from build123d import *

# Parameters (mm, degrees)
SKETCH1_W           = 33.5
SKETCH1_H           = 16
BOSS_EXTRUDE1_DEPTH = 32
SKETCH2_W           = 23.5
SKETCH2_H           = 16
CUT_EXTRUDE1_DEPTH  = 12
SKETCH4_R           = 0.5
BOSS_EXTRUDE2_DEPTH = 0.5
FILLET1_R           = 0.5
SKETCH6_W           = 16
SKETCH6_H           = 2
BOSS_EXTRUDE3_DEPTH = 75.5
SKETCH7_W           = 5
SKETCH7_H           = 5.252635659
CUT_EXTRUDE2_DEPTH  = 9
SKETCH8_R           = 0.8
CUT_EXTRUDE3_DEPTH  = 8
SKETCH9_R           = 0.5
SKETCH9_R_2         = 2
CUT_EXTRUDE4_DEPTH  = 8
FILLET2_R           = 30


with BuildPart() as part:
    # Sketch1 → Boss-Extrude1 (new body)
    with BuildSketch(Plane(origin=(0, 0, 0), x_dir=(1, 0, 0), z_dir=(0, 1, 0))):
        Rectangle(SKETCH1_W, SKETCH1_H)
    extrude(amount=BOSS_EXTRUDE1_DEPTH)

    # Sketch2 → Cut-Extrude1 (cut)
    with BuildSketch(Plane(origin=(0, 32, 0), x_dir=(1, 0, 0), z_dir=(0, 1, 0))):
        Rectangle(SKETCH2_W, SKETCH2_H)
    extrude(amount=-CUT_EXTRUDE1_DEPTH, mode=Mode.SUBTRACT)

    # Sketch4 → Boss-Extrude2 (add)
    with BuildSketch(Plane(origin=(0, 0, 0), x_dir=(-1, 0, 0), z_dir=(0, -1, 0))):
        with Locations(Location((15.81324072, -7.12248893, 0), (0, 0, 270))):
            Circle(SKETCH4_R)
        with Locations(Location((-15.868829232, -7.12248893, 0), (0, 0, 270))):
            Circle(SKETCH4_R)
        with Locations(Location((-15.868829232, 7.12248893, 0), (0, 0, 270))):
            Circle(SKETCH4_R)
        with Locations(Location((15.81324072, 7.12248893, 0), (0, 0, 270))):
            Circle(SKETCH4_R)
    extrude(amount=BOSS_EXTRUDE2_DEPTH)

    # Fillet1
    fillet1_edges = [part.edges().sort_by_distance(p)[0] for p in [
        (-15.81324072, -0.5, 6.62248893),
        (15.868829232, -0.5, 6.62248893),
        (15.868829232, -0.5, -7.62248893),
        (-15.81324072, -0.5, -7.62248893),
    ]]
    fillet(fillet1_edges, radius=FILLET1_R - 0.0001)  # a hair under: the kernel refuses the full size

    # Sketch6 → Boss-Extrude3 (add)
    with BuildSketch(Plane.ZY.offset(16.75)):
        with Locations((0, 31)):
            Rectangle(SKETCH6_W, SKETCH6_H)
    extrude(amount=BOSS_EXTRUDE3_DEPTH)

    # Sketch7 → Cut-Extrude2 (cut)
    with BuildSketch(Plane(origin=(0, 32, 0), x_dir=(1, 0, 0), z_dir=(0, 1, 0))):
        with Locations((14.25, -5.373682171)):
            Rectangle(SKETCH7_W, SKETCH7_H)
    extrude(amount=-CUT_EXTRUDE2_DEPTH, mode=Mode.SUBTRACT)

    # Sketch8 → Cut-Extrude3 (cut)
    with BuildSketch(Plane.XY):
        with Locations((13.65, 26)):
            Circle(SKETCH8_R)
        with Locations((-13.65, 26)):
            Circle(SKETCH8_R)
    extrude(amount=-CUT_EXTRUDE3_DEPTH, mode=Mode.SUBTRACT)

    # Sketch9 → Cut-Extrude4 (cut)
    with BuildSketch(Plane(origin=(0, 32, 0), x_dir=(1, 0, 0), z_dir=(0, 1, 0))):
        with Locations(Location((-88.515974664, 6.5, 0), (0, 0, 270))):
            Circle(SKETCH9_R)
        with Locations(Location((-75.25, 0, 0), (0, 0, 270))):
            Circle(SKETCH9_R)
        with Locations(Location((-88.515974664, -6.5, 0), (0, 0, 270))):
            Circle(SKETCH9_R)
        with Locations(Location((-88.515974664, 0, 0), (0, 0, 270))):
            Circle(SKETCH9_R_2)
    extrude(amount=-CUT_EXTRUDE4_DEPTH, mode=Mode.SUBTRACT)

    # Fillet2
    fillet2_edges = [part.edges().sort_by_distance(p)[0] for p in [
        (-16.75, 30, 0),
    ]]
    fillet(fillet2_edges, radius=FILLET2_R - 0.0001)  # a hair under: the kernel refuses the full size


solid = part.part
Input: part model. Units: mm. Frame: model coordinates. A direction names the side the tool comes from. Coordinates: 2 decimals unless noted, no trailing zeros. Loops run counter-clockwise (first coordinate to the right, second up) from the corner with the lowest first, then second, coordinate; pieces in that order, holes last.
(1) Material intervals for probe 1 along X at (y, z) = (31.3, 0); probe 2 along X at (y, z) = (31.5, -6.5); probe 3 along X at (y, z) = (31, 6.5), sorted ascending.
(2) Pull-direction query (X, two-part tool) for faces 1 (the face through (0, 20, 0)), 2 (the face through (-25.771, 21.445, 0.112)), 3 (the face through (14, 32, -3)); classes: released by +X, released by -X, zero draft, split by the parting line, or undercut.
(3) First-contact query: pin 1 Ø8 at (y, z) = (27.5, -3.5) entering from -X; pin 2 Ø5 at (x, z) = (-88.52, 0) entering from -Y; pin 3 Ø1 at (x, y) = (13.65, 26) entering from -Z; pin 4 Ø4 at (y, z) = (24.5, 1) entering from -X. Flat tips, straight axial feed; report the tip coordinate or a pass-through.
(4) Section C-C on y = 18.5. Return the cut outline in (x, z), then the cut area to 3 significant figures.
(5) Set-up query: faces 4 (the face through (14, 23, 5)), 5 (the face through (11.75, 26, -2)), 6 (the face through (-9, 17, -8)), 7 (the face through (16.75, 16, 0)), 8 (the face through (-69, 30, 0)). Return all of +Z, -Z, +X, -X, +Y, -Y with unobstructed straight access to the full face (end or side cutting, diameter ignored); none if empty.
(6) Section B-B on x = -72. Return the cut outline in (y, z).
Data:
1. probe 1: x = -92.25 to -90.52, -86.52 to -75.75, -74.75 to -11.75, 11.75 to 16.75
1. probe 2: x = -92.25 to -89.02, -88.02 to -11.75, 11.75 to 16.75
1. probe 3: x = -92.25 to -89.02, -88.02 to -11.75
2. face 1: undercut
2. face 2: released by -X
2. face 3: zero draft
3. pin 1: stops at x = -92.25
3. pin 2: stops at y = 30
3. pin 3: stops at z = 0
3. pin 4: stops at x = -32.69
4. outline: (-23.13, -8) - (16.75, -8) - (16.75, 8) - (-23.13, 8) - close
4. area: 638 mm2
5. face 4: +Z, +X, +Y
5. face 5: +Z, -Z, +Y
5. face 6: -Z, +X, -X, +Y, -Y
5. face 7: +Z, -Z, +X, +Y, -Y
5. face 8: +Z, -Z, -X, -Y
6. outline: (30, -8) - (32, -8) - (32, 8) - (30, 8) - close
